Part print with two shaded views. Sizes in mm from the minimum x, y, z corner. Give positions to 0.01 mm unless a question says otherwise; leave off trailing zeros. Order: outer loops, then holes, each group sorted by start corner. A loop starts at its lowest first (then second) coordinate and runs counter-clockwise, first axis right, second up. Notation, with made-up numbers: M -7.5,66 L 41.5,66 A20 cw 41.5,90 Z; hole C -17,53.5 d7. An arc over 180 degrees is marked long. Return JSON: item names as keys, results as strings. Group by question number.
1. Two-plate mould, pull along X, no slides. Class the marked faces 1, 2 and 3: released by +X, released by -X, zero draft, split by the parting line, or undercut.
2. Slice it at C-C on z = 2.8. List the corners of the cut face in (x, y), then the cut area to 3 significant figures.
3. Slice it at A-A on y = 3.25. List the corners of the cut face in (x, z).
4. Pin check, flat tips, straight feed: pin 1 (1 mm diameter, centred on x = 4, y = 4, fed in from +Z); pin 2 (2 mm diameter, centred on x = 2, z = 2.5, fed in from +Y); pin 3 (1 mm diameter, centred on x = 5, z = 3.5, fed in from -Y); pin 4 (1.5 mm diameter, centred on x = 4, y = 4.5, fed in from +Z). Stop position of each tip, or through.
5. Wall check: probe 1 along Y at (x, z) = (3.25, 1); probe 2 along Z at (x, y) = (1.75, 5.25); probe 3 along X at (y, z) = (2, 2.1). Give the ranges that are in metal, low to high. Write a range as [from, to].
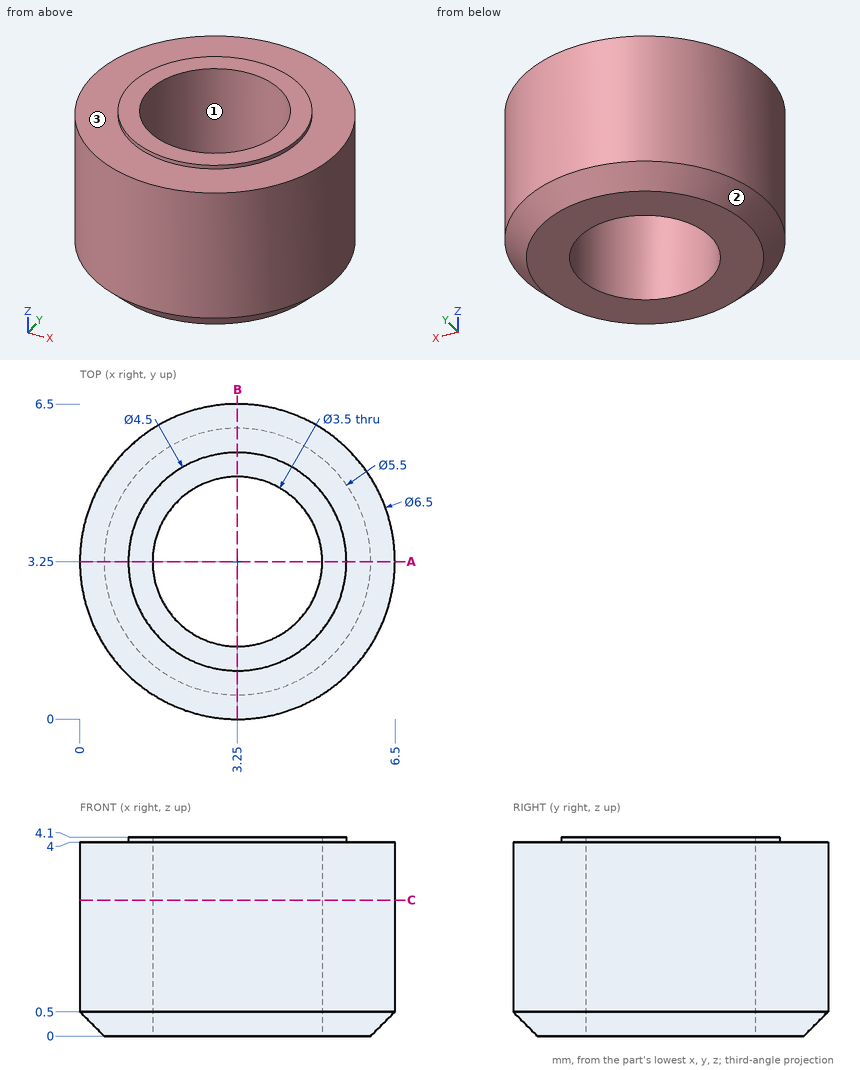
Result:
{
 "1": {"face 1": "undercut", "face 2": "split by the parting line", "face 3": "zero draft"},
 "2": {"outline": "C 3.25,3.25 d6.5; hole C 3.25,3.25 d3.5", "area": "23.6 mm2"},
 "3": {"outline": "M 0,0.5 L 0.5,0 L 1.5,0 L 1.5,4.1 L 1,4.1 L 1,4 L 0,4 Z; M 5,0 L 6,0 L 6.5,0.5 L 6.5,4 L 5.5,4 L 5.5,4.1 L 5,4.1 Z"},
 "4": {"pin 1": "passes through", "pin 2": "stops at y = 6.49", "pin 3": "stops at y = 0.25", "pin 4": "stops at z = 4.1"},
 "5": {"probe 1": "y = [0, 1.5], [5, 6.5]", "probe 2": "z = [0, 4]", "probe 3": "x = [0.25, 2.03], [4.47, 6.25]"}
}
